The figure shows three views and two pictorial views of one solid part (mm, origin at its lowest corner). Answer the questions. Round coordinates to 2 decimals unless told otherwise and drop trailing zeros. Order: outer loops, then holes, each group sorted by start corner. A loop starts at its lowest first (then second) coordinate and runs counter-clockwise, first axis right, second up. Notation, with made-up numbers: (-3.75, -27) - (41.25, -27) arc R24 ccw to (41.25, -16) - close; hole circle Ø10 at (18, 5.25). An arc over 180 degrees is marked (long way). One line per item, written item: value. Start each with the question number.
1. Section D-D, the plane x = 87.5 is taken. Give the vertices of the cut face in (y, z), then the cut area to 3 significant figures.
2. Section A-A, the plane z = 6 is taken. Give the vertices of the cut face in (x, y).
3. Flat-ended cylindrical pins translate along their axes: P1, Ø1.5, axis at x = 96.5, y = 2, coming from the -Z side; P2, Ø2.5, axis at x = 79, y = 1.5, coming from the +Z side; P3, Ø2.5, axis at y = 3, z = 73.5, coming from the +X side. Find the tip coordinate at first contact, or state that the pin passes through.
4. Section C-C, the plane x = 10 is taken. Give the vertices of the cut face in (y, z).
5. Straight lines are drawn through the part: line 1 (Z direction, x = 10, y = 1); line 2 (X direction, y = 1.8, z = 6); line 3 (Z direction, x = 69.5, y = 1.05). For each, find the intervals that lie inside material, in ascending order.
6. Section B-B, the plane y = 4 is taken. Give the vertices of the cut face in (x, z).
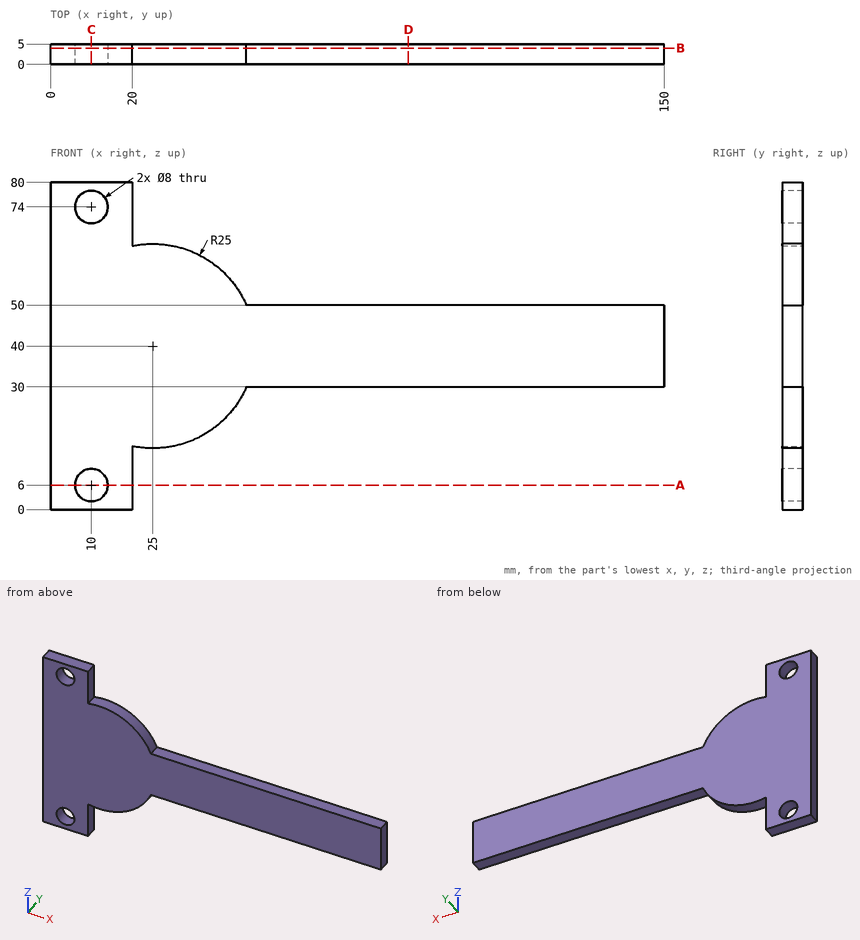
Answer list:
1. outline: (0, 30) - (5, 30) - (5, 50) - (0, 50) - close
1. area: 100 mm²
2. outline: (0, 0) - (6, 0) - (6, 5) - (0, 5) - close; (14, 0) - (20, 0) - (20, 5) - (14, 5) - close
3. P1: stops at z = 30
3. P2: stops at z = 50
3. P3: stops at x = 20
4. outline: (0, 0) - (5, 0) - (5, 2) - (0, 2) - close; (0, 10) - (5, 10) - (5, 70) - (0, 70) - close; (0, 78) - (5, 78) - (5, 80) - (0, 80) - close
5. line 1: z = 0 to 2, 10 to 70, 78 to 80
5. line 2: x = 0 to 6, 14 to 20
5. line 3: z = 30 to 50
6. outline: (0, 0) - (20, 0) - (20, 15.51) arc R25 ccw to (47.91, 30) - (150, 30) - (150, 50) - (47.91, 50) arc R25 ccw to (20, 64.49) - (20, 80) - (0, 80) - close; hole circle Ø8 at (10, 6); hole circle Ø8 at (10, 74)
